Here's the drawing with two shaded views (mm, measured from the low corner). I have some questions. A direction names the side the tool comes from. Round coordinates to 2 decimals unless told otherwise and drop trailing zeros. Order: outer loops, then holes, each group sorted by start corner. A loop starts at its lowest first (then second) coordinate and runs counter-clockwise, first axis right, second up. Notation, with made-up numbers: (-24, -28.75) -> (25, -28.75) arc R23 ccw to (25, -9.75) -> close; hole circle Ø7 at (38.5, -28.75). An arc over 180 degrees is marked (long way). One line per question, with ' | ' between items.
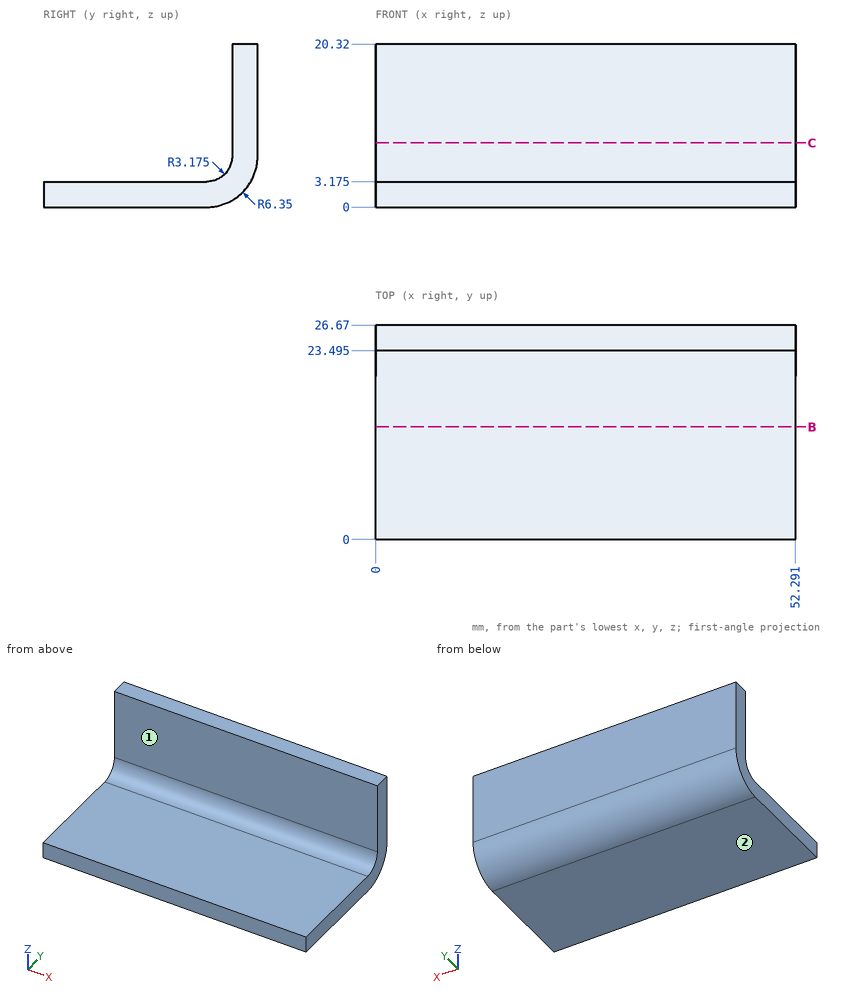
1. I'm going to push flat-ended pins straight in: pin 1 (8 mm diameter, centred on y = 12.5, z = 9, fed in from +X); pin 2 (1 mm diameter, centred on x = 12, z = 14, fed in from -Y) (3 decimals); pin 3 (10 mm diameter, centred on x = 10.5, y = 5.5, fed in from +Z) (3 decimals); pin 4 (3 mm diameter, centred on x = 12, z = 7, fed in from -Y). Where does each tip first touch, or does it pass through?
From the geometry:
pin 1: passes through | pin 2: stops at y = 23.495 | pin 3: stops at z = 3.175 | pin 4: stops at y = 23.38
2. I want a section at C-C on z = 8. List the corners of the cut face in (x, y) for me (1 decimal).
From the geometry:
outline: (0, 23.5) -> (52.3, 23.5) -> (52.3, 26.7) -> (0, 26.7) -> close
3. I need wall thicknesses on probe 1 along Y at (x, z) = (43, 12.25) (1 decimal); probe 2 along Z at (x, y) = (5.5, 20.5); probe 3 along Y at (x, z) = (14, 3.5) (1 decimal). Which ranges of each line are inside material? Lowest first, please.
From the geometry:
probe 1: y = 23.5 to 26.7 | probe 2: z = 0 to 3.18 | probe 3: y = 21.7 to 26
4. I want a section at B-B on y = 14. List the corners of the cut face in (x, z) for me (1 decimal).
From the geometry:
outline: (0, 0) -> (52.3, 0) -> (52.3, 3.2) -> (0, 3.2) -> close
5. On a 3-axis mill with a long thin cutter (end or side, diameter ignored), from which of +Z, -Z, +X, -X, +Y, -Y can I reach the whole of each face in a straight line? I mean the marked faces 1 and 2. Say none if no direction works.
From the geometry:
face 1: +Z, +X, -X, -Y | face 2: -Z, +X, -X, +Y, -Y
